```python
from build123d import *

# Parameters (mm, degrees)
SKETCH_W     = 184
SKETCH_H     = 100
PAD_DEPTH    = 100
SKETCH001_W  = 84.5
SKETCH001_H  = 90
POCKET_DEPTH = 95
FILLET_R     = 2


with BuildPart() as part:
    # Sketch → Pad (new body)
    with BuildSketch(Plane.XY):
        Rectangle(SKETCH_W, SKETCH_H)
    extrude(amount=PAD_DEPTH)

    # Sketch001 (on Face6 of Pad) → Pocket (cut)
    with BuildSketch(Plane.XY.offset(100)):
        with Locations((-44.75, 0)):
            Rectangle(SKETCH001_W, SKETCH001_H)
        with Locations((44.75, 0)):
            Rectangle(SKETCH001_W, SKETCH001_H)
    extrude(amount=-POCKET_DEPTH, mode=Mode.SUBTRACT)

    # Fillet
    fillet_edges = [part.edges().sort_by_distance(p)[0] for p in [
        (-92, 50, 50),
        (-92, -50, 50),
        (-92, 0, 0),
        (-92, 0, 100),
        (92, 50, 50),
        (0, 50, 0),
        (0, 50, 100),
        (92, -50, 50),
        (0, -50, 0),
        (0, -50, 100),
        (92, 0, 0),
        (92, 0, 100),
        (-87, 0, 100),
        (-44.75, -45, 100),
        (-2.5, 0, 100),
        (-44.75, 45, 100),
        (2.5, 0, 100),
        (44.75, -45, 100),
        (87, 0, 100),
        (44.75, 45, 100),
        (-87, 45, 52.5),
        (-87, -45, 52.5),
        (-87, 0, 5),
        (-2.5, -45, 52.5),
        (-44.75, -45, 5),
        (-2.5, 45, 52.5),
        (-2.5, 0, 5),
        (-44.75, 45, 5),
        (2.5, 45, 52.5),
        (2.5, -45, 52.5),
        (2.5, 0, 5),
        (87, -45, 52.5),
        (44.75, -45, 5),
        (87, 45, 52.5),
        (87, 0, 5),
        (44.75, 45, 5),
    ]]
    fillet(fillet_edges, radius=FILLET_R)


solid = part.part
```
The model under review builds one solid part; all positions refer to its coordinate system, in mm. A direction names the side the tool comes from. Give positions to 0.01 mm unless a question says otherwise; leave off trailing zeros. Write each loop counter-clockwise with the first axis right and the second up, starting at its lowest first coordinate (ties: lowest second). Pieces come first, ordered by that corner, then holes. Notation, with made-up numbers: M -22,32 L -3,32 A12 cw -3,37 Z; hole C 67.25,55.5 d9. An arc over 180 degrees is marked long. Write each question's results on one line, items separated by ' | '. Start each with the question number.
1. Mouldability with a two-part tool opening along X and no side actions: class faces 1 (the flat face through (44, 1, 5)), 2 (the flat face through (87, -1, 53)), 3 (the flat face through (-1, 1, 0)), 4 (the flat face through (92, -1, 49)) as released by +X, released by -X, zero draft, split by the parting line, or undercut.
2. We need section B-B (y = -14.5). Write out the cut boundary in (x, z), and give its area (3 significant figures).
3. We need section C-C (x = -35.5). Write out the cut boundary in (y, z), and give its area (3 significant figures).
4. We need section A-A (z = 35.5). Write out the cut boundary in (x, y).
5. For faces 5 (the flat face through (-87, -1, 53)), 6 (the flat face through (0, 0, 100)), list the 3-axis set-ups (+Z, -Z, +X, -X, +Y, -Y) from which the entire face can be reached by the end or side of a thin tool; tool diameter is ignored.
6. For probe 1 along X at (y, z) = (-29.5, 44.5); probe 2 along Y at (x, z) = (-69, 81); probe 3 along X at (y, z) = (43.5, 35.5), list the stretches that pass through material, from the lowest coordinate up. Write a range as [from, to].
Results found:
1) face 1: undercut | face 2: undercut | face 3: zero draft | face 4: released by +X
2) outline: M -92,2 A2 ccw -90,0 L 90,0 A2 ccw 92,2 L 92,98 A2 ccw 90,100 L 89,100 A2 ccw 87,98 L 87,7 A2 cw 85,5 L 4.5,5 A2 cw 2.5,7 L 2.5,98 A2 ccw 0.5,100 L -0.5,100 A2 ccw -2.5,98 L -2.5,7 A2 cw -4.5,5 L -85,5 A2 cw -87,7 L -87,98 A2 ccw -89,100 L -90,100 A2 ccw -92,98 Z | area: 2,340 mm^2
3) outline: M -50,2 A2 ccw -48,0 L 48,0 A2 ccw 50,2 L 50,98 A2 ccw 48,100 L 47,100 A2 ccw 45,98 L 45,7 A2 cw 43,5 L -43,5 A2 cw -45,7 L -45,98 A2 ccw -47,100 L -48,100 A2 ccw -50,98 Z | area: 1,450 mm^2
4) outline: M -92,-48 A2 ccw -90,-50 L 90,-50 A2 ccw 92,-48 L 92,48 A2 ccw 90,50 L -90,50 A2 ccw -92,48 Z; hole M -87,-43 A2 ccw -85,-45 L -4.5,-45 A2 ccw -2.5,-43 L -2.5,43 A2 ccw -4.5,45 L -85,45 A2 ccw -87,43 Z; hole M 2.5,-43 A2 ccw 4.5,-45 L 85,-45 A2 ccw 87,-43 L 87,43 A2 ccw 85,45 L 4.5,45 A2 ccw 2.5,43 Z
5) face 5: +Z | face 6: +Z, +X, -X, +Y, -Y
6) probe 1: x = [-92, -87], [-2.5, 2.5], [87, 92] | probe 2: y = [-50, -45], [45, 50] | probe 3: x = [-92, -86.94], [-2.56, 2.56], [86.94, 92]
